Source: CAD feature listing. Evaluate the final solid. Frame: model axes, mm. A direction names the side the tool comes from. Round coordinates to 2 decimals unless told otherwise and drop trailing zeros. Loops run counter-clockwise (first coordinate to the right, second up) from the corner with the lowest first, then second, coordinate; pieces in that order, holes last. Notation, with made-up numbers: M -20.5,-40 L 1.5,-40 A22 ccw 1.5,-29 Z; hole C -29.5,67.5 d1. An arc over 180 degrees is marked long. One line per item, written item: value.
Autodesk Inventor part; units mm, degrees
ref_plane "YZ Plane" through (0, 0, 0) normal (1, 0, 0) x (0, 1, 0)
ref_plane "XZ Plane" through (0, 0, 0) normal (0, 1, 0) x (-1, 0, 0)
ref_plane "XY Plane" through (0, 0, 0) normal (0, 0, 1) x (1, 0, 0)
sketch "Sketch1" plane through (0, 0, 0) normal (0, 0, 1) x (1, 0, 0)
  line L0 (-169.6995, 150.4778) -> (135.1005, 150.4778)
  line L1 (135.1005, 150.4778) -> (135.1005, -154.3222)
  line L2 (135.1005, -154.3222) -> (-169.6995, -154.3222)
  line L3 (-169.6995, -154.3222) -> (-169.6995, 150.4778)
  point P0 (0, 0)
  dimension "d0" = 304.8
extrude "Extrusion1" add sketch "Sketch1" along normal blind 2.9972
sketch "Sketch2" plane through (0, 0, 2.9972) normal (0, 0, 1) x (1, 0, 0)
  line L0 (135.1005, 150.4778) -> (-169.6995, 150.4778)
  line L1 (135.1005, -154.3222) -> (135.1005, 150.4778)
  line L2 (-169.6995, 150.4778) -> (135.1005, 150.4778)
  line L3 (135.1005, 150.4778) -> (135.1005, 147.4806)
  line L4 (135.1005, 147.4806) -> (-169.6995, 147.4806)
  line L5 (-169.6995, 147.4806) -> (-169.6995, 150.4778)
  point P0 (0, 0)
  dimension "d3" = 2.9972
extrude "Extrusion2" add sketch "Sketch2" along normal blind 301.8028
sketch "Sketch3" plane through (-169.6995, 150.4778, 0) normal (0, 1, 0) x (1, 0, 0)
  circle A0 centre (279.4, -139.7) radius 1.7272
  circle A1 centre (279.4, -152.4) radius 1.7272
  circle A2 centre (279.4, -165.1) radius 1.7272
  line L0 (279.4, -137.0931) -> (279.4, -150.7928) construction
  line L1 (304.8, 0) -> (304.8, -304.8)
  line L2 (304.8, -304.8) -> (0, -304.8)
  point P0 (169.6995, 0)
  dimension "d6" = 3.4544
  dimension "d7" = 12.7
  dimension "d8" = 12.7
  dimension "d9" = 25.4
  dimension "d10" = 152.4
extrude "Extrusion3" cut sketch "Sketch3" against normal through all
properties part number "Frame Test for Papa John"
1. Section query C-C (y = 112.5). Return the cut outline in (x, z), and give its area (3 significant figures).
Report:
outline: M -169.7,0 L 135.1,0 L 135.1,3 L -169.7,3 Z
area: 914 mm2
2. Ray query, line 1 (X direction, y = 149.6, z = 152.4); line 2 (Z direction, x = -89, y = -83); line 3 (Y direction, x = -20.5, z = 100). Return the intervals inside material, ascending. Write a range as [from, to].
Report:
line 1: x = [-169.7, 107.97], [111.43, 135.1]
line 2: z = [0, 3]
line 3: y = [147.48, 150.48]
3. Section query B-B (z = 133). Return the cut outline in (x, y).
Report:
outline: M -169.7,147.48 L 135.1,147.48 L 135.1,150.48 L -169.7,150.48 Z
4. Section query A-A (x = -75). Return the cut outline in (y, z).
Report:
outline: M -154.32,0 L 150.48,0 L 150.48,304.8 L 147.48,304.8 L 147.48,3 L -154.32,3 Z
5. Reachability of faces 1 (the face through (-19, 150.478, 150)), 2 (the face through (-19, -1, 2.997)) from +Z, -Z, +X, -X, +Y, -Y: full face, straight path, thin tool, end or side. Return the list, or none.
Report:
face 1: +Z, -Z, +X, -X, +Y
face 2: +Z, +X, -X, -Y
6. Pin query (flat end, axial travel): pin 1 (10 mm diameter, centred on x = -22, y = 45, fed in from -Z); pin 2 (2 mm diameter, centred on x = 109.7, z = 152.4, fed in from +Y); pin 3 (1 mm diameter, centred on x = -94.5, z = 97, fed in from -Y); pin 4 (12 mm diameter, centred on x = 20, y = -107, fed in from +Z). Return the tip coordinate at first contact, or that it passes through.
Report:
pin 1: stops at z = 0
pin 2: passes through
pin 3: stops at y = 147.48
pin 4: stops at z = 3
